Autodesk Inventor part; units mm, degrees
ref_plane "Work Plane2" through (0, 0, 5) normal (0, 0, 1) x (1, 0, 0)
ref_plane "Work Plane8" through (0, 0, 0) normal (0.8660254, 0.5, 0) x (0, 0, 1)
ref_plane "Work Plane9" through (0, 0, 0) normal (1, 0, 0) x (0, 1, 0)
sketch "Sketch1" plane through (0, 0, 0) normal (0, 0, 1) x (1, 0, 0)
  circle A0 centre (0, 0) radius 7.8659
  dimension "d0" = 15.7318
extrude "Extrusion1" add sketch "Sketch1" along normal blind 10
ref_plane "Work Plane2" through (0, 0, 5) normal (0, 0, 1) x (1, 0, 0)
sketch "Sketch2" plane through (0, 0, 0) normal (0, 0, -1) x (-1, 0, 0)
  circle A0 centre (0, 0) radius 7.8659
  circle A1 centre (0, 0) radius 6
  dimension "d3" = 12
surface extrude "Pitch Diameter" sketch "Sketch2" against normal through all shown no curves A1
ref_plane "Work Plane8" through (0, 0, 0) normal (0.8660254, 0.5, 0) x (0, 0, 1)
ref_plane "Work Plane9" through (0, 0, 0) normal (1, 0, 0) x (0, 1, 0)
spur gear teeth "Spur Gear" teeth 6 pitch diameter 12 tip diameter 15.7318 root diameter 7 face width 10 start plane through (0, 0, 0) normal (0, 0, -1) x (-1, 0, 0)
equation "\"d0\" = da_da"
equation "\"d1\" = da_b"
equation "\"d3\" = da_d"
properties part number "Spur Gear1" material "Steel"
Work out the finished part from the listing and answer in its coordinate system (mm). A direction names the side the tool comes from. Round coordinates to 2 decimals unless told otherwise and drop trailing zeros. Write each loop counter-clockwise with the first axis right and the second up, starting at its lowest first coordinate (ties: lowest second). Pieces come first, ordered by that corner, then holes.
1) A cutting plane is placed at C-C on z = 1.5. Determine the outline of the cut face in (x, y), and give its area (3 significant figures).
2) Determine the mould class of faces 6 (the face through (5.6, 1.45, 4.93)), 7 (the face through (0, 0, 0)), 8 (the face through (0.014, -7.866, 4.93)), 9 (the face through (1.546, 5.574, 4.93)) for opening direction Y: pulls with the +Y half, pulls with the -Y half, needs draft (parallel to the pull), parting line crosses it, or undercut.
3) Flat-ended cylindrical pins translate along their axes: P1, Ø6, axis at y = 2.5, z = 3, coming from the -X side; P2, Ø1.5, axis at y = -1, z = 2, coming from the -X side; P3, Ø1.5, axis at y = 5, z = 1.5, coming from the -X side. Find the tip coordinate at first contact, or state that the pin passes through.
4) Consider probe 1 along X at (y, z) = (-4, 9); probe 2 along Y at (x, z) = (4.75, 1); probe 3 along Y at (x, z) = (4.25, 6). Determine where each line is inside the solid, lowest interval first.
5) A cutting plane is placed at A-A on y = -4. Determine the outline of the cut face in (x, z), and give its area (3 significant figures).
6) Which of the six approach directions +Z, -Z, +X, -X, +Y, -Y give full straight-line access (tool end or side, diameter ignored) to faces 1 (the face through (-6.8, -3.95, 4.93)), 2 (the face through (-5.6, -1.45, 4.93)), 3 (the face through (4.054, -4.126, 4.93)), 4 (the face through (-4.054, 4.126, 4.93)), 5 (the face through (-1.55, 5.51, 4.93))?
7) A cutting plane is placed at B-B on x = 5.25. Determine the outline of the cut face in (y, z), and give its area (3 significant figures).
8) A cutting plane is placed at D-D on y = 4.5. Determine the outline of the cut face in (x, z).
Entries:
1. outline: (-7.27, -3.01) arc R7.87 ccw to (-6.24, -4.79) arc R7.33 ccw to (-2.13, -2.78) arc R3.5 ccw to (-1.34, -3.23) arc R7.33 ccw to (-1.03, -7.8) arc R7.87 ccw to (1.03, -7.8) arc R7.33 ccw to (1.34, -3.23) arc R3.5 ccw to (2.13, -2.78) arc R7.33 ccw to (6.24, -4.79) arc R7.87 ccw to (7.27, -3.01) arc R7.33 ccw to (3.47, -0.46) arc R3.5 ccw to (3.47, 0.46) arc R7.33 ccw to (7.27, 3.01) arc R7.87 ccw to (6.24, 4.79) arc R7.33 ccw to (2.13, 2.78) arc R3.5 ccw to (1.34, 3.23) arc R7.33 ccw to (1.03, 7.8) arc R7.87 ccw to (-1.03, 7.8) arc R7.33 ccw to (-1.34, 3.23) arc R3.5 ccw to (-2.13, 2.78) arc R7.33 ccw to (-6.24, 4.79) arc R7.87 ccw to (-7.27, 3.01) arc R7.33 ccw to (-3.47, 0.46) arc R3.5 ccw to (-3.47, -0.46) arc R7.33 ccw to start
1. area: 114 mm2
2. face 6: undercut
2. face 7: needs draft
2. face 8: pulls with the -Y half
2. face 9: undercut
3. P1: stops at x = -7.27
3. P2: stops at x = -6.01
3. P3: stops at x = -6.62
4. probe 1: x = -6.77 to -3.81, -1.49 to 1.49, 3.81 to 6.77
4. probe 2: y = -4.42 to -0.95, 0.95 to 4.42
4. probe 3: y = -4.22 to -0.72, 0.72 to 4.22
5. outline: (-6.77, 0) - (-3.81, 0) - (-3.81, 10) - (-6.77, 10) - close; (-1.49, 0) - (1.49, 0) - (1.49, 10) - (-1.49, 10) - close; (3.81, 0) - (6.77, 0) - (6.77, 10) - (3.81, 10) - close
5. area: 89.2 mm2
6. face 1: +Z, -Z, -X, -Y
6. face 2: +Z, -Z, -X
6. face 3: +Z, -Z, -Y
6. face 4: +Z, -Z, +Y
6. face 5: +Z, -Z
7. outline: (-4.58, 0) - (-1.22, 0) - (-1.22, 10) - (-4.58, 10) - close; (1.22, 0) - (4.58, 0) - (4.58, 10) - (1.22, 10) - close
7. area: 67.1 mm2
8. outline: (-6.45, 0) - (-4.98, 0) - (-4.98, 10) - (-6.45, 10) - close; (-1.55, 0) - (1.55, 0) - (1.55, 10) - (-1.55, 10) - close; (4.98, 0) - (6.45, 0) - (6.45, 10) - (4.98, 10) - close
